Can you work these out from the model? Positions are in its coordinate system, mm. A direction names the side the tool comes from. Coordinates: 2 decimals unless noted, no trailing zeros. Loops run counter-clockwise (first coordinate to the right, second up) from the corner with the lowest first, then second, coordinate; pieces in that order, holes last. Notation, with made-up numbers: (75.5, 26.5) -> (94.5, 26.5) arc R17 cw to (94.5, 59.5) -> close; hole circle Ø3 at (15, 13). An arc over 180 degrees is marked (long way). Put each result on its own line as item: value. Start each with the question number.
Item 1: Please list where these lines run through material, in increasing order: L1, parallel to Y at x = 9, z = 0 (3 decimals); L2, parallel to Y at x = 29, z = 0 (3 decimals); L3, parallel to Z at x = 20, y = -0.5. Write a range as from..to.
Item 2: If we section it at A-A on y = 0: Please give me the cut outline in (x, z) (3 decimals).
Item 3: If we section it at C-C on y = 20: State how many separate pieces and enclosed holes the cut face has, plus the area to 3 significant figures.
Item 4: Will these pins go through, and if not, where does the flat tip stop? P1, Ø1.6, axis at y = -12, z = 0, coming from the -X side; P2, Ø12, axis at x = 4.5, z = -3, coming from the +Y side; P3, Ø5, axis at x = 15.5, z = 1, coming from the +Y side.
Item 5: For faces 4 (the cylindrical face through (1.425, 18.536, 0.325)), 5 (the conical face through (4.812, 13.724, 7.138)), which set-ups out of +Z, -Z, +X, -X, +Y, -Y let a thin tool reach every point of the face, with its end or its side?
Item 6: We'd pull the mould along Z, two halves only. Please class faces 1 (the cylindrical face through (15.21, 13.363, 0.179)), 2 (the flat face through (0, 0, 5)), 3 (the cylindrical face through (28.986, 19.961, 10.382)): pulls with the +Z half, pulls with the -Z half, needs draft (parallel to the pull), parting line crosses it, or undercut.
Item 7: If we section it at B-B on x = 6.5: Please give me the cut outline in (y, z) (3 decimals).
```python
from build123d import *

# Parameters (mm, degrees)
SKETCH2_R          = 1.375
SKETCH2_R_2        = 1.5
CUT_EXTRUDE1_DEPTH = 44.732139211


with BuildPart() as part:
    # Sketch1 → Revolve1 (revolve)
    with BuildSketch(Plane(origin=(0, 0, 0), x_dir=(1, 0, 0), z_dir=(0, 1, 0)), mode=Mode.PRIVATE) as revolve1_sk:
        Polygon((5, 15), (2, 22.5), (0, 22.5), (0, 3.25), (30, 3.25), (30, 22.5), (28, 22.5), (24.995890376, 15), align=None)
    revolve(revolve1_sk.sketch.rotate(Axis((0, 0, 0), (1, 0, 0)), 180), axis=Axis((0, 0, 0), (1, 0, 0)))

    # Sketch2 → Cut-Extrude1 (cut, through all)
    with BuildSketch(Plane(origin=(30, 0, 0), x_dir=(0, 0, -1), z_dir=(1, 0, 0))):
        with Locations((0, 12)):
            Circle(SKETCH2_R)
        with Locations((0, 20)):
            Circle(SKETCH2_R_2)
        with Locations((12, 0)):
            Circle(SKETCH2_R)
        with Locations((0, -12)):
            Circle(SKETCH2_R)
        with Locations((-12, 0)):
            Circle(SKETCH2_R)
    extrude(amount=-CUT_EXTRUDE1_DEPTH, mode=Mode.SUBTRACT)


solid = part.part
```
Solutions:
1. L1: -15..-13.375, -10.625..-3.25, 3.25..10.625, 13.375..15
1. L2: -22.5..-13.375, -10.625..-3.25, 3.25..10.625, 13.375..18.5, 21.5..22.5
1. L3: -14.99..-13.28, -10.72..-3.21, 3.21..10.72, 13.28..14.99
2. outline: (0, -22.5) -> (2, -22.5) -> (5, -15) -> (24.996, -15) -> (28, -22.5) -> (30, -22.5) -> (30, -13.375) -> (0, -13.375) -> close; (0, -10.625) -> (30, -10.625) -> (30, -3.25) -> (0, -3.25) -> close; (0, 3.25) -> (30, 3.25) -> (30, 10.625) -> (0, 10.625) -> close; (0, 13.375) -> (30, 13.375) -> (30, 22.5) -> (28, 22.5) -> (24.996, 15) -> (5, 15) -> (2, 22.5) -> (0, 22.5) -> close
3. separate pieces: 4
3. enclosed holes: 0
3. area: 91.7 mm^2
4. P1: through
4. P2: y = 22.5
4. P3: y = 15
5. face 4: +X, -X
5. face 5: none
6. face 1: undercut
6. face 2: needs draft
6. face 3: parting line crosses it
7. outline: circle Ø30 at (0, 0); hole circle Ø2.75 at (-12, 0); hole circle Ø6.5 at (0, 0); hole circle Ø2.75 at (0, -12); hole circle Ø2.75 at (0, 12); hole circle Ø2.75 at (12, 0)
